```python
from build123d import *

# Parameters (mm, degrees)
BASE_PLATE_DEPTH     = 2
M3_CLEARANCE_HOLE1_D = 3.4
FILLET1_R            = 3


with BuildPart() as part:
    # Sketch1 → Base Plate (new body)
    with BuildSketch(Plane.XY):
        Polygon((31.8, 0), (-31.8, 0), (-31.8, -29), (-45, -29), (-45, -69), (45, -69), (45, -29), (31.8, -29), align=None)
    extrude(amount=BASE_PLATE_DEPTH)

    # M3 Clearance Hole1 (through all)
    with Locations(Plane.XY.offset(2)):
        with Locations((-23.4, -7), (-8.4, -7), (-8.4, -22), (-23.4, -22), (-33.3, -61), (33.3, -61), (8.4, -22), (23.4, -22), (8.4, -7), (23.4, -7)):
            Hole(M3_CLEARANCE_HOLE1_D / 2)

    # Fillet1
    fillet1_edges = [part.edges().sort_by_distance(p)[0] for p in [
        (31.8, -29, 1),
        (-31.8, -29, 1),
    ]]
    fillet(fillet1_edges, radius=FILLET1_R)


solid = part.part
```
CAD build for the part. Positions are in the model's coordinates, mm. A direction names the side the tool comes from. Round coordinates to 2 decimals unless told otherwise and drop trailing zeros. Write each loop counter-clockwise with the first axis right and the second up, starting at its lowest first coordinate (ties: lowest second). Pieces come first, ordered by that corner, then holes.
Item 1: Tool access for faces 1 (the flat face through (-1, -69, 1)), 2 (the flat face through (-40, -29, 1)): list every direction of +Z, -Z, +X, -X, +Y, -Y with a clear straight run to the whole face (end or side of a thin tool).
Filled in:
face 1: +Z, -Z, +X, -X, -Y
face 2: +Z, -Z, -X, +Y
Item 2: Mould opens along X. For faces 3 (the cylindrical face through (25.1, -6.93, 0.99)), 4 (the flat face through (31.8, -13, 1)), 5 (the cylindrical face through (-24.97, -7.65, 0.99)), 6 (the flat face through (0, 0, 1)) say: released by +X, released by -X, zero draft, split by the parting line, or undercut.
Filled in:
face 3: undercut
face 4: released by +X
face 5: undercut
face 6: zero draft
Item 3: Drill centre lines: L1, parallel to Y at x = 8.4, z = 1.1; L2, parallel to Y at x = 22.5, z = 0.75; L3, parallel to X at y = -8, z = 1.05. Where is each one in solid material? Low to high.
Filled in:
L1: y = -69 to -23.7, -20.3 to -8.7, -5.3 to 0
L2: y = -69 to -23.44, -20.56 to -8.44, -5.56 to 0
L3: x = -31.8 to -24.77, -22.03 to -9.77, -7.03 to 7.03, 9.77 to 22.03, 24.77 to 31.8
Item 4: Band-saw the part on D-D on x = -33.3. Write the cut outline in (y, z).
Filled in:
outline: (-69, 0) - (-62.7, 0) - (-62.7, 2) - (-69, 2) - close; (-59.3, 0) - (-28.6, 0) - (-28.6, 2) - (-59.3, 2) - close
Item 5: Band-saw the part on A-A on y = -7. Write the cut outline in (x, z).
Filled in:
outline: (-31.8, 0) - (-25.1, 0) - (-25.1, 2) - (-31.8, 2) - close; (-21.7, 0) - (-10.1, 0) - (-10.1, 2) - (-21.7, 2) - close; (-6.7, 0) - (6.7, 0) - (6.7, 2) - (-6.7, 2) - close; (10.1, 0) - (21.7, 0) - (21.7, 2) - (10.1, 2) - close; (25.1, 0) - (31.8, 0) - (31.8, 2) - (25.1, 2) - close
Item 6: Drop flat-ended pins along their axis: pin 1 Ø1 at (x, z) = (-39, 0.5) entering from +Y; pin 2 Ø0.6 at (y, z) = (-18.5, 0.5) entering from +X. Give the stop position or say it passes through.
Filled in:
pin 1: stops at y = -29
pin 2: stops at x = 31.8
Item 7: Band-saw the part on C-C on x = 8.4. Write the cut outline in (y, z), then the cut area to 3 significant figures.
Filled in:
outline: (-69, 0) - (-23.7, 0) - (-23.7, 2) - (-69, 2) - close; (-20.3, 0) - (-8.7, 0) - (-8.7, 2) - (-20.3, 2) - close; (-5.3, 0) - (0, 0) - (0, 2) - (-5.3, 2) - close
area: 124 mm2
Item 8: Band-saw the part on B-B on z = 0.95. Give the number of separate pieces and of enclosed holes in the cut face, then the cut area to 3 significant figures.
Filled in:
separate pieces: 1
enclosed holes: 10
area: 5,360 mm2
